from build123d import *

# Parameters (mm, degrees)
F0_W     = 18
F0_H     = 12
F0_R     = 3.5
F1_DEPTH = 15
F2_SIZE  = 3
F3_SIZE  = 1
F4_SIZE  = 0.5


with BuildPart() as f1:
    # F0 (on Top) → F1 (new body)
    with BuildSketch(Plane.XY):
        Rectangle(F0_W, F0_H)
        with Locations((0, -1)):
            Circle(F0_R, mode=Mode.SUBTRACT)
    extrude(amount=F1_DEPTH)

    # F2
    f2_edges = [f1.edges().sort_by_distance(p)[0] for p in [
        (9, -6, 7.5),
        (-9, -6, 7.5),
    ]]
    chamfer(f2_edges, length=F2_SIZE)

    # F3
    f3_edges = [f1.edges().sort_by_distance(p)[0] for p in [
        (9, 6, 7.5),
        (-9, 6, 7.5),
    ]]
    chamfer(f3_edges, length=F3_SIZE)

    # F4
    f4_edges = [f1.edges().sort_by_distance(p)[0] for p in [
        (-3.5, -1, 0),
        (-3.5, -1, 15),
    ]]
    chamfer(f4_edges, length=F4_SIZE)


solid = f1.part
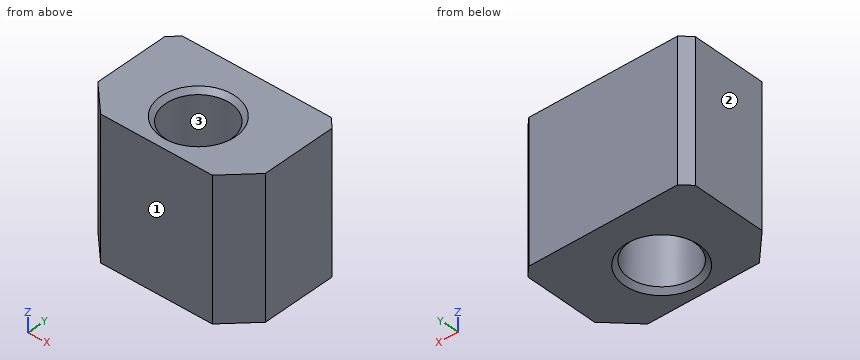
Here's how the part is built. I have some questions about the finished solid (model axes, mm). Face numbers are marked on the shaded views. Coordinates: 2 decimals unless noted, no trailing zeros. Order: outer loops, then holes, each group sorted by start corner. A loop starts at its lowest first (then second) coordinate and runs counter-clockwise, first axis right, second up. Notation, with made-up numbers: (75, 26.5) -> (122, 26.5) arc R17 ccw to (122, 42.5) -> close; hole circle Ø10 at (-14, 31.25). An arc over 180 degrees is marked (long way). Answer in a Markdown table with one row per item.
(1) I want a section at B-B on x = 0. List the corners of the cut face in (y, z) for me.
Answer key:
| item | result |
|---|---|
| outline | (-6, 0) -> (-5, 0) -> (-4.5, 0.5) -> (-4.5, 14.5) -> (-5, 15) -> (-6, 15) -> close; (2.5, 0.5) -> (3, 0) -> (6, 0) -> (6, 15) -> (3, 15) -> (2.5, 14.5) -> close |
(2) I want a section at D-D on x = 6.25. List the corners of the cut face in (y, z) for me, then the cut area to 3 significant figures.
Answer key:
| item | result |
|---|---|
| outline | (-5.75, 0) -> (6, 0) -> (6, 15) -> (-5.75, 15) -> close |
| area | 176 mm^2 |
(3) Thinking about a two-plate mould opening in X: for the marked faces 1, 2 and 3, which applies, +X half, -X half, draft (parallel to the pull), parting line (faces both ways), or undercut?
Answer key:
| item | result |
|---|---|
| face 1 | draft |
| face 2 | -X half |
| face 3 | undercut |
(4) Please list where these lines run through material, in increasing order: probe 1 along Y at (x, z) = (0, 4.25); probe 2 along Y at (x, z) = (-3, 4.75); probe 3 along Y at (x, z) = (-7, 0.5).
Answer key:
| item | result |
|---|---|
| probe 1 | -6 to -4.5, 2.5 to 6 |
| probe 2 | -6 to -2.8, 0.8 to 6 |
| probe 3 | -5 to 6 |
(5) I want a section at C-C on z = 8.75. List the corners of the cut face in (x, y) for me, then the cut area to 3 significant figures.
Answer key:
| item | result |
|---|---|
| outline | (-9, -3) -> (-6, -6) -> (6, -6) -> (9, -3) -> (9, 5) -> (8, 6) -> (-8, 6) -> (-9, 5) -> close; hole circle Ø7 at (0, -1) |
| area | 168 mm^2 |
(6) I want a section at A-A on y = -1. List the corners of the cut face in (x, z) for me.
Answer key:
| item | result |
|---|---|
| outline | (-9, 0) -> (-4, 0) -> (-3.5, 0.5) -> (-3.5, 14.5) -> (-4, 15) -> (-9, 15) -> close; (3.5, 0.5) -> (4, 0) -> (9, 0) -> (9, 15) -> (4, 15) -> (3.5, 14.5) -> close |
